The model under review builds one solid part; all positions refer to its coordinate system, in mm. Face numbers are marked on the shaded views. Give positions to 0.01 mm unless a question says otherwise; leave off trailing zeros. Loops run counter-clockwise (first coordinate to the right, second up) from the corner with the lowest first, then second, coordinate; pieces in that order, holes last. Notation, with made-up numbers: M -15,-31.75 L 2,-31.75 A3 cw 2,-26.75 Z; hole C -36,89 d8. An arc over 180 degrees is marked long. Return JSON: item names as keys, results as strings.
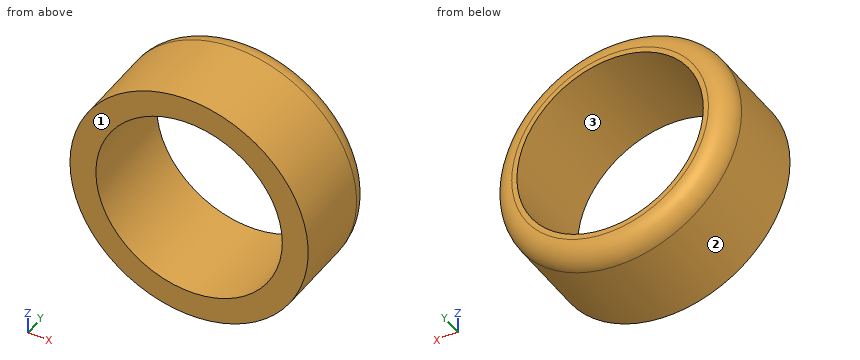
Autodesk Inventor part; units mm, degrees
ref_plane "YZ Plane" through (0, 0, 0) normal (1, 0, 0) x (0, 1, 0)
ref_plane "XZ Plane" through (0, 0, 0) normal (0, 1, 0) x (-1, 0, 0)
ref_plane "XY Plane" through (0, 0, 0) normal (0, 0, 1) x (1, 0, 0)
sketch "Sketch2" plane through (0, 0, 0) normal (0, 1, 0) x (-1, 0, 0)
  circle A0 centre (0, 0) radius 11.5
  dimension "d2" = 23
extrude "Extrusion1" add sketch "Sketch2" along normal blind 9.8
sketch "Sketch3" plane through (0, 9.8, 0) normal (0, 1, 0) x (1, 0, 0)
  circle A0 centre (0, 0) radius 9
  dimension "d5" = 18
extrude "Extrusion2" cut sketch "Sketch3" against normal through all
fillet "Fillet1" radius 2 1 edges at (11.5, 9.8, 0)
properties part number "Tires"
1) Consider section C-C on y = 5.75. Write out the cut boundary in (x, z), then the cut area to 3 significant figures.
From the geometry:
{"outline": "C 0,0 d23; hole C 0,0 d18", "area": "161 mm²"}
2) Wall thickness on L1, parallel to Z at x = 0, y = 7.25; L2, parallel to X at y = 5.25, z = -7; L3, parallel to X at y = 1.5, z = -1.75: over which ranges is each line inside the solid? List them lowest first. Write a range as from..to.
From the geometry:
{"L1": "-11.5..-9, 9..11.5", "L2": "-9.12..-5.66, 5.66..9.12", "L3": "-11.37..-8.83, 8.83..11.37"}
3) The part is to be moulded in two halves that separate along Z. For the marked faces 1, 2 and 3, say which applies: released by +Z, released by -Z, zero draft, split by the parting line, or undercut.
From the geometry:
{"face 1": "zero draft", "face 2": "split by the parting line", "face 3": "undercut"}
4) Consider section A-A on z = 0. Write out the cut boundary in (x, y).
From the geometry:
{"outline": "M -11.5,0 L -9,0 L -9,9.8 L -9.5,9.8 A2 ccw -11.5,7.8 Z; M 9,0 L 11.5,0 L 11.5,7.8 A2 ccw 9.5,9.8 L 9,9.8 Z"}
5) Consider section B-B on x = 0. Write out the cut boundary in (y, z), then the cut area to 3 significant figures.
From the geometry:
{"outline": "M 0,-11.5 L 7.8,-11.5 A2 ccw 9.8,-9.5 L 9.8,-9 L 0,-9 Z; M 0,9 L 9.8,9 L 9.8,9.5 A2 ccw 7.8,11.5 L 0,11.5 Z", "area": "47.3 mm²"}
6) Insertion check: pin 1 (1.5 mm diameter, centred on y = 7.5, z = 2, fed in from -X); pin 2 (3 mm diameter, centred on y = 2, z = 2.5, fed in from -X); pin 3 (4 mm diameter, centred on x = -5.5, y = 5, fed in from +Z); pin 4 (4 mm diameter, centred on x = 2.5, z = -5, fed in from +Y). Each pin has a flat end and moves straight along its axis. Give the tip position at first contact, or say it passes through.
From the geometry:
{"pin 1": "x = -11.43", "pin 2": "x = -11.46", "pin 3": "z = 10.95", "pin 4": "through"}
